Geometry: final body of the model. Coordinates: model frame, mm. A direction names the side the tool comes from. Round coordinates to 2 decimals unless told otherwise and drop trailing zeros. Loops run counter-clockwise (first coordinate to the right, second up) from the corner with the lowest first, then second, coordinate; pieces in that order, holes last. Notation, with made-up numbers: M 48.5,16 L 56.5,16 A27 cw 56.5,51 Z; hole C 61.25,-1 d10. An arc over 180 degrees is marked long. Return JSON: item names as keys, results as strings.
Autodesk Inventor part; units mm, degrees
ref_plane "YZ Plane" through (0, 0, 0) normal (1, 0, 0) x (0, 1, 0)
ref_plane "XZ Plane" through (0, 0, 0) normal (0, 1, 0) x (-1, 0, 0)
ref_plane "XY Plane" through (0, 0, 0) normal (0, 0, 1) x (1, 0, 0)
sketch "Sketch1" plane through (0, 0, 0) normal (0, 1, 0) x (-1, 0, 0)
  line L0 (0, -16) -> (0, -22)
  line L1 (0, -22) -> (4.5992, -22)
  arc A0 (7.5587, -25.4914) -> (4.5992, -22) centre (4.5992, -25) ccw
  arc A1 (7.5587, -25.4914) -> (10.6423, -30.0525) centre (11.5046, -26.1465) ccw
  arc A2 (18.0009, -55.917) -> (11.9694, -31.0524) centre (-31.9884, -54.8791) ccw
  arc A3 (18.0009, -55.917) -> (22, -60) centre (22, -56) ccw
  line L2 (22, -60) -> (28, -60)
  arc A4 (28, -60) -> (28.9223, -52.1078) centre (28, -56) ccw
  line L3 (27.5709, -51.0069) -> (23.1874, -41.6064)
  line L4 (23.0076, -40.9355) -> (19.4262, 0)
  arc A5 (11.9694, -31.0524) -> (10.6423, -30.0525) centre (10.2111, -32.0054) ccw
  line L5 (0, -16) -> (6, -16)
  line L6 (10, -12) -> (10, 0)
  arc A6 (6, -16) -> (10, -12) centre (6, -12) ccw
  arc A7 (22.2903, -50.042) -> (12.4, -27.35) centre (-30.8395, -59.6973) ccw
  line L7 (28, -56) -> (42.0245, -56)
  line L8 (22.2903, -50.042) -> (35.4778, -47.6454)
  line L9 (-30.8395, -59.6973) -> (22.2903, -50.042)
  line L10 (-30.8395, -59.6973) -> (12.4, -27.35)
  circle A8 centre (22.2903, -50.042) radius 1.5
  circle A9 centre (21.1713, -45.1756) radius 1.5
  circle A10 centre (19.6075, -40.4334) radius 1.5
  circle A11 centre (17.6125, -35.856) radius 1.5
  circle A12 centre (15.2031, -31.4824) radius 1.5
  circle A13 centre (12.4, -27.35) radius 1.5
  circle A14 centre (5.5, -19) radius 1.5
  circle A15 centre (10, -19) radius 1.5
  circle A16 centre (18.5, -19) radius 1.5
  circle A17 centre (11.5, -23.5) radius 1.5
  circle A18 centre (28, -56) radius 1.5
  circle A19 centre (22, -56) radius 1.5
  arc A20 (23.0076, -40.9355) -> (23.1874, -41.6064) centre (25, -40.7612) ccw
  arc A21 (27.5709, -51.0069) -> (28.9223, -52.1078) centre (29.3835, -50.1617) ccw
  line L11 (19.4262, 0) -> (10, 0)
  point P0 (0, 0)
  point P1 (28.0341, -52.0001)
  dimension "d0" = 28
  dimension "d1" = 0
  dimension "d2" = 2
  dimension "d3" = 4
  dimension "d4" = 12
  dimension "d5" = 0
  dimension "d6" = 10
  dimension "d8" = 5
  dimension "d9" = 20
  dimension "d10" = 4
  dimension "d11" = 4
  dimension "d12" = 50
  dimension "d13" = 4
  dimension "d14" = 3
  dimension "d15" = 54
  dimension "d16" = 10.3
  dimension "d17" = 26.5
  dimension "d18" = 27.35
  dimension "d19" = 12.4
  dimension "d20" = 3
  dimension "d21" = 56
  dimension "d22" = 0
  dimension "d25" = 26.5
  dimension "d28" = 3
  dimension "d29" = 3
  dimension "d30" = 3
  dimension "d31" = 5.5
  dimension "d32" = 4.5
  dimension "d34" = 19
  dimension "d35" = 3
  dimension "d36" = 4.5
  dimension "d38" = 13
  dimension "d39" = 3
  dimension "d40" = 6
  dimension "d42" = 3
  dimension "d43" = 3
  dimension "d44" = 2
extrude "Extrusion2" add sketch "Sketch1" along normal blind 3 contours L5 A6 L6 L11 L4 A20 L3 L8 A8 A7 A9 A10 A11 A12 A13 L10 A1 A0 L1 L0 | L10 A13 A7 A12 A11 A10 A9 A8 L9 A2 A5 A1 | L9 A8 L8 L3 A21 A4 L2 A3 A2
mirror "Mirror1" about plane through (-19.4262, 0, 0) normal (0, 0, 1) of "Extrusion2"
properties part number "500-120"
Q1. Pin query (flat end, axial travel): pin 1 (2.5 mm diameter, centred on x = -11.5, z = -23.5, fed in from +Y) (1 decimal). Return the tip coordinate at first contact, or that it passes through.
Determined:
{"pin 1": "passes through"}
Q2. Section query D-D (y = 2.3). State how many separate pieces and enclosed holes the cut face has, plus the area to 3 significant figures.
Determined:
{"separate pieces": "1", "enclosed holes": "24", "area": "1,210 mm^2"}
Q3. Material intervals for L1, parallel to Z at x = -13.5, y = 1.1; L2, parallel to Z at x = -6, y = 2; L3, parallel to Z at x = -12.4, y = 0.8, sorted ascending.
Determined:
{"L1": "z = -34.12 to -28.37, -26.33 to 26.33, 28.37 to 34.12", "L2": "z = -22.35 to -20.41, -17.59 to -16, 16 to 17.59, 20.41 to 22.35", "L3": "z = -31.86 to -28.85, -25.85 to -24.7, -22.3 to 22.3, 24.7 to 25.85, 28.85 to 31.86"}
Q4. Section query B-B (z = 23.5). Output: boundary loops of the cut face in (x, y).
Determined:
{"outline": "M -21.48,0 L -13,0 L -13,3 L -21.48,3 Z; M -10,0 L -7.2,0 L -7.2,3 L -10,3 Z"}
Q5. Reachability of faces 1 (the cylindrical face through (-8.797, 1.479, 14.859)), 2 (the cylindrical face through (-11.305, 1.479, -24.987)), 3 (the flat face through (-25.41, 1.48, -46.37)), 4 (the flat face through (-2, 1, 22)) from +Z, -Z, +X, -X, +Y, -Y: full face, straight path, thin tool, end or side. Return the list, or none.
Determined:
{"face 1": "+X, +Y, -Y", "face 2": "+Y, -Y", "face 3": "-X, +Y, -Y", "face 4": "+Z, +X, +Y, -Y"}
Q6. Pull-direction query (X, two-part tool) for faces 5 (the cylindrical face through (-26.5, 1.48, 55.93)), 6 (the flat face through (0, 1, -19)), 7 (the flat face through (-21.19, 1.48, 20.18)); classes: pulls with the +X half, pulls with the -X half, needs draft (parallel to the pull), parting line crosses it, or undercut.
Determined:
{"face 5": "undercut", "face 6": "pulls with the +X half", "face 7": "pulls with the -X half"}
Q7. Section query C-C (z = 6). Output: boundary loops of the cut face in (x, y).
Determined:
{"outline": "M -19.95,0 L -10,0 L -10,3 L -19.95,3 Z"}
Q8. Section query A-A (x = -2.5). Output: boundary loops of the cut face in (y, z), plus the area to 3 significant figures.
Determined:
{"outline": "M 0,-22 L 3,-22 L 3,-16 L 0,-16 Z; M 0,16 L 3,16 L 3,22 L 0,22 Z", "area": "36.0 mm^2"}
